from build123d import *

# Parameters (mm, degrees)
SKETCH1_W           = 45
SKETCH1_H           = 20
SKETCH1_R           = 8
SKETCH1_H_2         = 13
SKETCH1_H_3         = 1
BOSS_EXTRUDE1_DEPTH = 3
SKETCH3_W           = 45
SKETCH3_H           = 2.9
SKETCH3_H_2         = 6.2
BOSS_EXTRUDE2_DEPTH = 11.5
SKETCH3_3_W         = 45
SKETCH3_3_H         = 2.9
BOSS_EXTRUDE3_DEPTH = 21.5
SKETCH6_R           = 1.525
SKETCH6_W           = 10.1
SKETCH6_H           = 10
CUT_EXTRUDE2_DEPTH  = 16.5
CHAMFER1_SIZE       = 5
FILLET2_R           = 5
FILLET3_SIZE        = 7
FILLET3_SIZE_2      = 6
SKETCH7_R           = 0.996709825
SKETCH7_R_2         = 1
BOSS_EXTRUDE4_DEPTH = 3
CHAMFER2_SIZE       = 10
CHAMFER3_SIZE       = 10
CHAMFER4_START      = 17.731133084
CHAMFER4_DEPTH      = 3.699865449
CHAMFER5_START      = -16.752681828
CHAMFER5_DEPTH      = 1.71299366


with BuildPart() as part:
    # Sketch1 → Boss-Extrude1 (new body)
    # profile 1 of 3: a face of its own
    with BuildSketch(Plane(origin=(0, 0, 0), x_dir=(1, 0, 0), z_dir=(0, 1, 0))):
        Rectangle(SKETCH1_W, SKETCH1_H)
        with Locations(Location((13, 0, 0), (0, 0, 270))):
            Circle(SKETCH1_R, mode=Mode.SUBTRACT)
        with Locations(Location((-13, 0, 0), (0, 0, 270))):
            Circle(SKETCH1_R, mode=Mode.SUBTRACT)
    # profile 2 of 3: a face of its own
    with BuildSketch(Plane(origin=(0, 0, 0), x_dir=(1, 0, 0), z_dir=(0, 1, 0))):
        with Locations((0, -16.5)):
            Rectangle(SKETCH1_W, SKETCH1_H_2)
    # profile 3 of 3: a face of its own
    with BuildSketch(Plane(origin=(0, 0, 0), x_dir=(1, 0, 0), z_dir=(0, 1, 0))):
        with Locations((0, -10.5)):
            Rectangle(SKETCH1_W, SKETCH1_H_3)
    extrude(amount=BOSS_EXTRUDE1_DEPTH)

    # Sketch3 → Boss-Extrude2 (add)
    with BuildSketch(Plane(origin=(0, 3, 0), x_dir=(1, 0, 0), z_dir=(0, 1, 0))):
        with Locations((0, -21.55)):
            Rectangle(SKETCH3_W, SKETCH3_H)
        with Locations((0, -17)):
            Rectangle(SKETCH3_W, SKETCH3_H_2)
        with Locations((0, -12.45)):
            Rectangle(SKETCH3_W, SKETCH3_H)
    extrude(amount=BOSS_EXTRUDE2_DEPTH)

    # Sketch3<3> → Boss-Extrude3 (add)
    with BuildSketch(Plane(origin=(0, 3, 0), x_dir=(1, 0, 0), z_dir=(0, 1, 0))):
        with Locations((0, -12.45)):
            Rectangle(SKETCH3_3_W, SKETCH3_3_H)
        with Locations((0, -21.55)):
            Rectangle(SKETCH3_3_W, SKETCH3_3_H)
    extrude(amount=BOSS_EXTRUDE3_DEPTH)

    # Sketch6 → Cut-Extrude2 (cut)
    with BuildSketch(Plane(origin=(0, 0, 11), x_dir=(-1, 0, 0), z_dir=(0, 0, -1))):
        with Locations((-6.15, 19.5)):
            Circle(SKETCH6_R)
        with Locations((6.15, 19.5)):
            Circle(SKETCH6_R)
        with Locations((-17.45, 19.5)):
            Rectangle(SKETCH6_W, SKETCH6_H)
        with Locations((17.45, 19.5)):
            Rectangle(SKETCH6_W, SKETCH6_H)
    extrude(amount=-CUT_EXTRUDE2_DEPTH, mode=Mode.SUBTRACT)

    # Chamfer1
    chamfer1_edges = [part.edges().sort_by_distance(p)[0] for p in [
        (0, 0, 23),
    ]]
    chamfer(chamfer1_edges, length=CHAMFER1_SIZE)

    # Fillet2
    fillet2_edges = [part.edges().sort_by_distance(p)[0] for p in [
        (-22.5, 1.5, -10),
        (22.5, 1.5, -10),
    ]]
    fillet(fillet2_edges, radius=FILLET2_R)

    # Fillet3
    # a fillet whose section is not a circle: 7, 6 mm, written as the material it takes off along each edge
    with BuildSketch(Plane(origin=(12.4, 24.5, -6.5), x_dir=(-1, 0, 0), z_dir=(0, 0, 1)), Plane(origin=(-12.4, 24.5, -6.5), x_dir=(0, -1, 0), z_dir=(0, 0, 1))) as fillet3_piece_1:
        with BuildLine():
            Bezier((FILLET3_SIZE, 0), (0, 0), (0, FILLET3_SIZE_2), weights=[1, 0.707106781, 1])
            Line((0, FILLET3_SIZE_2), (0, 0))
            Line((0, 0), (FILLET3_SIZE, 0))
        make_face()
    extrude(amount=37.9, mode=Mode.SUBTRACT)
    with BuildSketch(Plane(origin=(12.4, 24.5, 2.6), x_dir=(0, -1, 0), z_dir=(0, 0, 1)), Plane(origin=(-12.4, 24.5, 2.6), x_dir=(1, 0, 0), z_dir=(0, 0, 1))) as fillet3_piece_2:
        with BuildLine():
            Bezier((FILLET3_SIZE_2, 0), (0, 0), (0, -FILLET3_SIZE), weights=[1, 0.707106781, 1])
            Line((0, -FILLET3_SIZE), (0, 0))
            Line((0, 0), (FILLET3_SIZE_2, 0))
        make_face()
    extrude(amount=37.9, mode=Mode.SUBTRACT)

    # Sketch7 → Boss-Extrude4 (add)
    with BuildSketch(Plane.XZ):
        with BuildLine():
            Line((-10, -10), (10, -10))
            Line((10, -10), (10, -18.132118098))
            Line((10, -18.132118098), (6.075, -18.132118098))
            Line((6.075, -18.132118098), (6.075, -15.047815402))
            ThreePointArc((6.075, -15.047815402), (4.848419821, -11.842215517), (1.689491671, -10.5))
            Line((1.689491671, -10.5), (-1.689458819, -10.5))
            ThreePointArc((-1.689458819, -10.5), (-4.736103523, -11.729921298), (-6.075, -14.730272374))
            Line((-6.075, -14.730272374), (-6.075, -18.132118098))
            Line((-6.075, -18.132118098), (-10, -18.132118098))
            Line((-10, -18.132118098), (-10, -10))
        make_face()
        with Locations(Location((8, -15, 0), (0, 0, 270))):
            Circle(SKETCH7_R, mode=Mode.SUBTRACT)
        with Locations(Location((-8, -15, 0), (0, 0, 270))):
            Circle(SKETCH7_R_2, mode=Mode.SUBTRACT)
    extrude(amount=-BOSS_EXTRUDE4_DEPTH)

    # Chamfer2
    # the kernel refuses this chamfer: 10 mm, written as the material it takes off along each edge
    with BuildSketch(Plane(origin=(22.5, 23.184544799, 41.184544799), x_dir=(0, 0.7071067811865476, -0.7071067811865476), z_dir=(0, -0.7071067811865476, -0.7071067811865476))) as chamfer2_piece_1:
        Polygon((CHAMFER2_SIZE, 0), (0, -CHAMFER2_SIZE), (0, 0), align=None)
    extrude(amount=58.504727571, mode=Mode.SUBTRACT)

    # Chamfer3
    # the kernel refuses this chamfer: 10 mm, written as the material it takes off along each edge
    with BuildSketch(Plane(origin=(-22.5, 23.184544799, 41.184544799), x_dir=(1, 0, 0), z_dir=(0, -0.7071067811865476, -0.7071067811865476))) as chamfer3_piece_1:
        Polygon((CHAMFER3_SIZE, 0), (0, -CHAMFER3_SIZE), (0, 0), align=None)
    extrude(amount=58.504727571, mode=Mode.SUBTRACT)

    # Chamfer4: read off the stored shape, not the designer's step
    # Chamfer4 outline → Chamfer4 (cut)
    with BuildSketch(Plane(origin=(0, 0, 0), x_dir=(0.3029024372169638, 0.9530210691127028, -0.0009774227869083028), z_dir=(0.9530161074355918, -0.302904014214538, -0.0030752464993570898)).offset(CHAMFER4_START)):
        Polygon((8.846062674, 11.063231546), (18.37626426, 11.072546631), (18.323534543, 16.02226833), align=None)
    extrude(amount=CHAMFER4_DEPTH, mode=Mode.SUBTRACT)

    # Chamfer5: read off the stored shape, not the designer's step
    # Chamfer5 outline → Chamfer5 (cut)
    with BuildSketch(Plane(origin=(0, 0, 0), x_dir=(-0.2371114626358165, 0.9695954628947141, -0.06052100974611115), z_dir=(0.9394753911891737, 0.24471337996518516, 0.2397943932121102)).offset(CHAMFER5_START)):
        Polygon((18.381427339, 16.222851439), (14.80832265, 19.648555484), (6.951420363, 15.508917831), align=None)
    extrude(amount=CHAMFER5_DEPTH, mode=Mode.SUBTRACT)


solid = part.part
Can you work these out from the model? Positions are in its coordinate system, mm. A direction names the side the tool comes from. Coordinates: 2 decimals unless noted, no trailing zeros. Write each loop counter-clockwise with the first axis right and the second up, starting at its lowest first coordinate (ties: lowest second). Pieces come first, ordered by that corner, then holes.
Q1. Imagine slicing it at D-D, the plane z = 16.5. List the corners of the cut face in (x, y) for me, plus the area to 3 significant figures.
Results found:
outline: (-22.5, 12.64) - (-13.56, 0) - (13.56, 0) - (22.5, 12.64) - (22.5, 14.5) - (-22.5, 14.5) - close
area: 539 mm2
Q2. Imagine slicing it at A-A, the plane z = 0. List the corners of the cut face in (x, y) for me, plus the area to 3 significant figures.
Results found:
outline: (-22.5, 0) - (-21, 0) - (-21, 3) - (-22.5, 3) - close; (-5, 0) - (5, 0) - (5, 3) - (-5, 3) - close; (21, 0) - (22.5, 0) - (22.5, 3) - (21, 3) - close
area: 39.0 mm2
Q3. For P1, Ø3.5, axis at x = 13.5, y = 1.5, coming from the -Z side; P2, Ø1.5, axis at y = 1.5, z = -17, coming from the +X side; P3, Ø1.5, axis at y = 2, z = -16, coming from the -X side, each with a flat end and sliding along its axis, tell me the tip position at first contact or that it passes through.
Results found:
P1: stops at z = -10
P2: stops at x = 10
P3: stops at x = -10
Q4. Which directions (+Z, -Z, +X, -X, +Y, -Y) give clear straight access to the entire face, cutting with the end or side of a thin tool? Please do faces 1 (the face through (-8, 1, -18.132)), 2 (the face through (-10, 1, -14)), 3 (the face through (10, 1, -14)), 4 (the face through (-6.075, 1, -16)), 5 (the face through (22.5, 13, 14)).
Results found:
face 1: -Z, +X, -X, +Y, -Y
face 2: -Z, -X, +Y, -Y
face 3: -Z, +X, +Y, -Y
face 4: -Z, +Y, -Y
face 5: +Z, -Z, +X, +Y, -Y
Q5. Imagine slicing it at C-C, the plane y = 4.25. List the corners of the cut face in (x, z) for me, plus the area to 3 significant figures.
Results found:
outline: (-20.06, 11.55) - (-19.92, 11) - (19.99, 11) - (19.99, 11.65) - (12.5, 22.25) - (-12.5, 22.25) - close
area: 370 mm2
Q6. Imagine slicing it at B-B, the plane x = 0.5. List the corners of the cut face in (y, z) for me, plus the area to 3 significant figures.
Results found:
outline: (0, -10.5) - (3, -10.5) - (3, 11) - (24.5, 11) - (24.5, 13.9) - (14.5, 13.9) - (14.5, 20.1) - (24.5, 20.1) - (24.5, 23) - (5, 23) - (0, 18) - close
area: 284 mm2
Q7. If we mould it in two halves opening along Z, with no side actions, what happens to faces 6 (the face through (-1, 24.5, 12)), 7 (the face through (21, 1.52, -8.57)), 8 (the face through (0, 15, 23)), 9 (the face through (0, 14.5, 17))? For each: +Z half, -Z half, draft (parallel to the pull), parting line (faces both ways), or undercut.
Results found:
face 6: draft
face 7: -Z half
face 8: +Z half
face 9: undercut
Q8. Please list where these lines run through material, in increasing order: L1, parallel to X at y = 1.75, z = 0; L2, parallel to Z at x = -3, y = 21; L3, parallel to X at y = 1.35, z = -15 (3 decimals).
Results found:
L1: x = -22.5 to -21, -5 to 5, 21 to 22.5
L2: z = 11 to 13.9, 20.1 to 23
L3: x = -10 to -9, -7 to -6.075, 6.076 to 7.003, 8.997 to 10
